from build123d import *

# Parameters (mm, degrees)
F0_R     = 8
F0_R_2   = 4.986346
F0_R_3   = 4.028364
F1_DEPTH = 2
F0_R_4   = 3
F2_DEPTH = 18
F3_R     = 4.986346
F4_DEPTH = 12
F5_DEPTH = 44.1
F6_SIZE  = 0.25
F7_SIZE  = 0.5


with BuildPart() as f1:
    # F0 (on Top) → F1 (new body)
    with BuildSketch(Plane.XY):
        Circle(F0_R)
        Circle(F0_R_2, mode=Mode.SUBTRACT)
        Circle(F0_R_2)
        Circle(F0_R_3, mode=Mode.SUBTRACT)
    extrude(amount=F1_DEPTH)

    # F0 (on Top) → F2 (join)
    with BuildSketch(Plane.XY):
        Circle(F0_R_4)
        Circle(F0_R_3)
        Circle(F0_R_4, mode=Mode.SUBTRACT)
    extrude(amount=F2_DEPTH)

    # F3 (on face) → F4 (join)
    with BuildSketch(Plane.XY.offset(18)):
        Circle(F3_R)
    extrude(amount=-F4_DEPTH)

    # F0 (on Top) → F5 (cut)
    with BuildSketch(Plane.XY):
        Circle(F0_R_4)
    extrude(amount=F5_DEPTH, mode=Mode.SUBTRACT)

    # F6
    f6_edges = [f1.edges().sort_by_distance(p)[0] for p in [
        (8, 0, 1),
        (-8, 0, 0),
        (-8, 0, 2),
    ]]
    chamfer(f6_edges, length=F6_SIZE)

    # F7
    f7_edges = [f1.edges().sort_by_distance(p)[0] for p in [
        (-4.986346, 0, 6),
        (-4.986346, 0, 18),
    ]]
    chamfer(f7_edges, length=F7_SIZE)


solid = f1.part
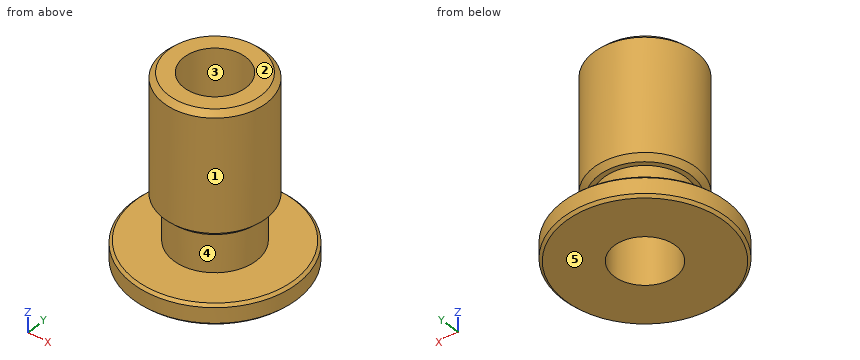
Read the model definition and answer for the solid it produces. Units are mm, in the model's axes. Face numbers are marked on the shaded views. A direction names the side the tool comes from. Round coordinates to 2 decimals unless told otherwise and drop trailing zeros. Order: outer loops, then holes, each group sorted by start corner. A loop starts at its lowest first (then second) coordinate and runs counter-clockwise, first axis right, second up. Notation, with made-up numbers: (12, 12.5) - (46, 12.5) arc R20 cw to (46, 32.5) - close; hole circle Ø7 at (69.5, 57). An arc over 180 degrees is marked (long way). Use one line per item in the form item = value. Start each with the question number.
(1) Flat-ended cylindrical pins translate along their axes: pin 1 Ø3 at (x, z) = (5.5, 13.5) entering from -Y; pin 2 Ø1 at (x, y) = (6, 0) entering from +Z; pin 3 Ø2.5 at (x, y) = (1, 0) entering from -Z; pin 4 Ø1 at (x, y) = (-5, -1) entering from +Z. Find the tip coordinate at first contact, or state that the pin passes through.
(2) Find the intervals of material crossed by line 1 along Y through (x, z) = (0, 11); line 2 along X through (y, z) = (0, 4.5), in increasing order. Write a range as from..to.
(3) The part is cut by section C-C (z = 7.5). Give the vertices of the cut face in (x, y).
(4) For the marked faces 1 and 2, determine the directions among +Z, -Z, +X, -X, +Y, -Y from which every point of the face is accessible in a straight line to the end or side of a thin tool.
(5) The part is cut by section A-A (x = 0). Give the vertices of the cut face in (y, z), then the cut area to 3 significant figures.
(6) Determine the mould class of the marked faces 3, 4 and 5 for opening direction X: +X half, -X half, draft (parallel to the pull), parting line (faces both ways), or undercut.
Checked values:
q1.pin_1 = -2.98
q1.pin_2 = 2
q1.pin_3 = through
q1.pin_4 = 17.89
q2.line_1 = -4.99..-3, 3..4.99
q2.line_2 = -4.03..-3, 3..4.03
q3.outline = circle Ø9.97 at (0, 0); hole circle Ø6 at (0, 0)
q4.face_1 = +Z
q4.face_2 = +Z, +X, -X, +Y, -Y
q5.outline = (-8, 0.25) - (-7.75, 0) - (-3, 0) - (-3, 18) - (-4.49, 18) - (-4.99, 17.5) - (-4.99, 6.5) - (-4.49, 6) - (-4.03, 6) - (-4.03, 2) - (-7.75, 2) - (-8, 1.75) - close; (3, 0) - (7.75, 0) - (8, 0.25) - (8, 1.75) - (7.75, 2) - (4.03, 2) - (4.03, 6) - (4.49, 6) - (4.99, 6.5) - (4.99, 17.5) - (4.49, 18) - (3, 18) - close
q5.area = 75.3 mm^2
q6.face_3 = undercut
q6.face_4 = parting line
q6.face_5 = draft
